```python
from build123d import *

# Parameters (mm, degrees)
SALIENTE_EXTRUIR1_DEPTH = 3
REDONDEO1_R             = 10
CROQUIS2_R              = 1.5
CROQUIS2_R_2            = 1.55
CORTAR_EXTRUIR1_DEPTH   = 135.610141171
CROQUIS4_W              = 110
CROQUIS4_H              = 50
CORTAR_EXTRUIR2_DEPTH   = 135.610141171
REDONDEO2_R             = 5
CROQUIS5_W              = 4
CROQUIS5_H              = 14.636342218
CORTAR_EXTRUIR3_DEPTH   = 135.610141171
CROQUIS6_W              = 14.636342218
CROQUIS6_H              = 3
SALIENTE_EXTRUIR2_DEPTH = 2
CROQUIS8_W              = 14.636342218
CROQUIS8_H              = 3
SALIENTE_EXTRUIR3_DEPTH = 2
CROQUIS9_W              = 196.2
CROQUIS9_H              = 31.087527503
CORTAR_EXTRUIR4_DEPTH   = 133.713564137
CROQUIS10_R             = 2
CORTAR_EXTRUIR5_DEPTH   = 133.713564137
REDONDEO6_R             = 15


with BuildPart() as part:
    # Croquis1 → Saliente-Extruir1 (new body)
    with BuildSketch(Plane(origin=(0, 0, 0), x_dir=(1, 0, 0), z_dir=(0, 1, 0))):
        Polygon((-88.1, 42.318171109), (88.1, 42.318171109), (108.1, 22.318171109), (127.75, 22.318171109), (127.75, 7.681828891), (105.75, 7.681828891), (77.75, -42.318171109), (-77.75, -42.318171109), (-105.75, 7.681828891), (-127.75, 7.681828891), (-127.75, 22.318171109), (-108.1, 22.318171109), align=None)
    extrude(amount=SALIENTE_EXTRUIR1_DEPTH)

    # Redondeo1
    redondeo1_edges = [part.edges().sort_by_distance(p)[0] for p in [
        (-88.1, 1.5, -42.318171109),
        (88.1, 1.5, -42.318171109),
        (108.1, 1.5, -22.318171109),
        (105.75, 1.5, -7.681828891),
        (77.75, 1.5, 42.318171109),
        (-77.75, 1.5, 42.318171109),
        (-105.75, 1.5, -7.681828891),
        (-108.1, 1.5, -22.318171109),
    ]]
    fillet(redondeo1_edges, radius=REDONDEO1_R)

    # Croquis2 → Cortar-Extruir1 (cut, through all)
    with BuildSketch(Plane(origin=(0, 3, 0), x_dir=(1, 0, 0), z_dir=(0, 1, 0))):
        with Locations(Location((70, -27.318171109, 0), (0, 0, 270))):
            Circle(CROQUIS2_R)
        with Locations(Location((-70, -27.318171109, 0), (0, 0, 270))):
            Circle(CROQUIS2_R)
        with Locations(Location((-119.996067812, 15, 0), (0, 0, 270))):
            Circle(CROQUIS2_R_2)
        with Locations(Location((119.996067812, 15, 0), (0, 0, 270))):
            Circle(CROQUIS2_R_2)
        with Locations(Location((-17.5, -17.318171109, 0), (0, 0, 270))):
            Circle(CROQUIS2_R)
        with Locations(Location((17.5, -17.318171109, 0), (0, 0, 270))):
            Circle(CROQUIS2_R)
        with Locations(Location((-17.5, -37.318171109, 0), (0, 0, 270))):
            Circle(CROQUIS2_R)
        with Locations(Location((17.5, -37.318171109, 0), (0, 0, 270))):
            Circle(CROQUIS2_R)
    extrude(amount=-CORTAR_EXTRUIR1_DEPTH, mode=Mode.SUBTRACT)

    # Croquis4 → Cortar-Extruir2 (cut, through all)
    with BuildSketch(Plane(origin=(0, 3, 0), x_dir=(1, 0, 0), z_dir=(0, 1, 0))):
        with Locations((0, -17.318171109)):
            Rectangle(CROQUIS4_W, CROQUIS4_H)
    extrude(amount=-CORTAR_EXTRUIR2_DEPTH, mode=Mode.SUBTRACT)

    # Redondeo2
    redondeo2_edges = [part.edges().sort_by_distance(p)[0] for p in [
        (55, 1.5, 42.318171109),
        (-55, 1.5, 42.318171109),
        (-55, 1.5, -7.681828891),
        (55, 1.5, -7.681828891),
    ]]
    fillet(redondeo2_edges, radius=REDONDEO2_R)

    # Croquis5 → Cortar-Extruir3 (cut, through all)
    with BuildSketch(Plane(origin=(0, 3, 0), x_dir=(1, 0, 0), z_dir=(0, 1, 0))):
        with Locations((-125.75, 15)):
            Rectangle(CROQUIS5_W, CROQUIS5_H)
        with Locations((125.75, 15)):
            Rectangle(CROQUIS5_W, CROQUIS5_H)
    extrude(amount=-CORTAR_EXTRUIR3_DEPTH, mode=Mode.SUBTRACT)

    # Croquis6 → Saliente-Extruir2 (add)
    with BuildSketch(Plane(origin=(123.75, 0, 0), x_dir=(0, 0, -1), z_dir=(1, 0, 0))):
        with Locations((15, 1.5)):
            Rectangle(CROQUIS6_W, CROQUIS6_H)
    extrude(amount=SALIENTE_EXTRUIR2_DEPTH)

    # Croquis8 → Saliente-Extruir3 (add)
    with BuildSketch(Plane.ZY.offset(123.75)):
        with Locations((-15, 1.5)):
            Rectangle(CROQUIS8_W, CROQUIS8_H)
    extrude(amount=SALIENTE_EXTRUIR3_DEPTH)

    # Croquis9 → Cortar-Extruir4 (cut, through all)
    with BuildSketch(Plane(origin=(0, 3, 0), x_dir=(1, 0, 0), z_dir=(0, 1, 0))):
        with Locations((0, 50.861934861)):
            Rectangle(CROQUIS9_W, CROQUIS9_H)
    extrude(amount=-CORTAR_EXTRUIR4_DEPTH, mode=Mode.SUBTRACT)

    # Croquis10 → Cortar-Extruir5 (cut, through all)
    with BuildSketch(Plane(origin=(0, 3, 0), x_dir=(1, 0, 0), z_dir=(0, 1, 0))):
        with Locations(Location((-52.5, 27.318171109, 0), (0, 0, 270))):
            Circle(CROQUIS10_R)
        with Locations(Location((52.5, 27.318171109, 0), (0, 0, 270))):
            Circle(CROQUIS10_R)
    extrude(amount=-CORTAR_EXTRUIR5_DEPTH, mode=Mode.SUBTRACT)

    # Redondeo6
    redondeo6_edges = [part.edges().sort_by_distance(p)[0] for p in [
        (-95.1, 1.5, -35.318171109),
        (95.1, 1.5, -35.318171109),
    ]]
    fillet(redondeo6_edges, radius=REDONDEO6_R)


solid = part.part
```
Can you work these out from the model? Positions are in its coordinate system, mm. A direction names the side the tool comes from. Coordinates: 2 decimals unless noted, no trailing zeros. Loops run counter-clockwise (first coordinate to the right, second up) from the corner with the lowest first, then second, coordinate; pieces in that order, holes last. Notation, with made-up numbers: (-32, 36.5) -> (-7, 36.5) arc R35 cw to (-7, 71.5) -> close; hole circle Ø2 at (-31, 28). An arc over 180 degrees is marked (long way). Put each result on its own line as item: value. Start each with the question number.
Q1. If I drill on line 1 (X direction, y = 2.1, z = -15); line 2 (Z direction, x = -70, y = 1.6); line 3 (X direction, y = 1.1, z = -26), over which ranges is the centre line in solid material (lowest first)? Write a range as [from, to].
Q2. I want a section at D-D (x = -91). Write out the boundary of the cut face in (y, z), plus the area to 3 significant figures.
Q3. For faces 1 (the face through (102.29, 1.48, -28.13)), 2 (the face through (-53.57, 1.48, -6.18)), which set-ups out of +Z, -Z, +X, -X, +Y, -Y let a thin tool reach every point of the face, with its end or its side?
Q4. I'm going to push flat-ended pins straight in: P1, Ø1.5, axis at x = 118, y = 2, coming from the +Z side; P2, Ø1.8, axis at x = -70, z = 27.32, coming from the +Y side; P3, Ø1.5, axis at y = 2, z = 10, coming from the -X side. Where does each tip first touch, or does it pass through?
Q5. I want a section at A-A (z = 2). Write out the boundary of the cut face in (x, y), plus the area to 3 significant figures.
Q6. I want a section at B-B (y = 1.6). Count the separate pieces of the cut face and the enclosed holes in it, plus the area to 3 significant figures.
Q7. I want a section at C-C (x = 94). Write out the boundary of the cut face in (y, z), plus the area to 3 significant figures.
Q8. Thinking about a two-plate mould opening in X: for faces 3 (the face through (53.496, 1.479, -6.256)), 4 (the face through (-56.5, 1.48, 40.89)), 5 (the face through (77.009, 1.521, 40.908)), 6 (the face through (-94.703, 1.521, -34.145)), which applies, pulls with the +X half, pulls with the -X half, needs draft (parallel to the pull), parting line crosses it, or undercut?
Taken from the geometry:
1. line 1: x = [-125.75, -121.55], [-118.45, 118.45], [121.55, 125.75]
1. line 2: z = [-35.32, 25.82], [28.82, 42.32]
1. line 3: x = [-104.42, -54], [-51, 51], [54, 104.42]
2. outline: (0, -35.17) -> (3, -35.17) -> (3, 18.66) -> (0, 18.66) -> close
2. area: 161 mm2
3. face 1: -Z, +X, +Y, -Y
3. face 2: +Z, +Y, -Y
4. P1: stops at z = -7.68
4. P2: passes through
4. P3: stops at x = -96.27
5. outline: (-100.33, 0) -> (-55, 0) -> (-55, 3) -> (-100.33, 3) -> close; (55, 0) -> (100.33, 0) -> (100.33, 3) -> (55, 3) -> close
5. area: 272 mm2
6. separate pieces: 1
6. enclosed holes: 6
6. area: 9,940 mm2
7. outline: (0, -34.42) -> (3, -34.42) -> (3, 13.3) -> (0, 13.3) -> close
7. area: 143 mm2
8. face 3: undercut
8. face 4: undercut
8. face 5: pulls with the +X half
8. face 6: pulls with the -X half
